from build123d import *

# Parameters (mm, degrees)
MODEL_R                 = 8
SALIENTE_EXTRUIR1_DEPTH = 3


with BuildPart() as part:
    # Model → Saliente-Extruir1 (new body)
    with BuildSketch(Plane.XY):
        with BuildLine():
            Line((25.103364369, 60.449776828), (25.103364369, 55.560048431))
            Line((25.103364369, 55.560048431), (25.103364369, -26.439158767))
            ThreePointArc((25.103364369, -26.439158767), (22.813551952, -32.073921627), (17.210031036, -34.439158767))
            Line((17.210031036, -34.439158767), (17.077324369, -34.439158767))
            Line((17.077324369, -34.439158767), (17.077324369, -36.439158767))
            Line((17.077324369, -36.439158767), (17.077324369, -37.439158767))
            Line((17.077324369, -37.439158767), (9.634620202, -37.439158767))
            ThreePointArc((9.634620202, -37.439158767), (8.940767121, -37.73835668), (8.658097702, -38.439105914))
            Line((8.658097702, -38.439105914), (8.658097702, -53.106951569))
            ThreePointArc((8.658097702, -53.106951569), (8.944324254, -53.811296927), (9.644764369, -54.106951569))
            Line((9.644764369, -54.106951569), (16.090657702, -54.106951569))
            ThreePointArc((16.090657702, -54.106951569), (16.791097817, -54.402606212), (17.077324369, -55.106951569))
            Line((17.077324369, -55.106951569), (17.077324369, -61.439951569))
            ThreePointArc((17.077324369, -61.439951569), (16.791097817, -62.144296927), (16.090657702, -62.439951569))
            Line((16.090657702, -62.439951569), (5.154444792, -62.439951569))
            Line((5.154444792, -62.439951569), (5.154444792, -58.439951569))
            Line((5.154444792, -58.439951569), (2.194444792, -58.439951569))
            Line((2.194444792, -58.439951569), (2.194444792, -62.439951569))
            Line((2.194444792, -62.439951569), (-2.852355631, -62.439951569))
            Line((-2.852355631, -62.439951569), (-2.852355631, -34.439951569))
            Line((-2.852355631, -34.439951569), (-11.074248964, -34.439951569))
            Line((-11.074248964, -34.439951569), (-11.074248964, -62.439951569))
            Line((-11.074248964, -62.439951569), (-15.565555208, -62.439951569))
            Line((-15.565555208, -62.439951569), (-15.565555208, -58.439951569))
            Line((-15.565555208, -58.439951569), (-18.525555208, -58.439951569))
            Line((-18.525555208, -58.439951569), (-18.525555208, -62.439951569))
            Line((-18.525555208, -62.439951569), (-30.017262298, -62.439951569))
            ThreePointArc((-30.017262298, -62.439951569), (-30.717702412, -62.144296927), (-31.003928964, -61.439951569))
            Line((-31.003928964, -61.439951569), (-31.003928964, -55.106951569))
            ThreePointArc((-31.003928964, -55.106951569), (-30.717702412, -54.402606212), (-30.017262298, -54.106951569))
            Line((-30.017262298, -54.106951569), (-23.571368964, -54.106951569))
            ThreePointArc((-23.571368964, -54.106951569), (-22.87092885, -53.811296927), (-22.584702298, -53.106951569))
            Line((-22.584702298, -53.106951569), (-22.584702298, -38.439951569))
            ThreePointArc((-22.584702298, -38.439951569), (-22.87092885, -37.735606212), (-23.571368964, -37.439951569))
            Line((-23.571368964, -37.439951569), (-31.003928964, -37.439951569))
            Line((-31.003928964, -37.439951569), (-31.003928964, -34.439951569))
            Line((-31.003928964, -34.439951569), (-31.136635631, -34.439951569))
            ThreePointArc((-31.136635631, -34.439951569), (-36.740156547, -32.074714429), (-39.029968964, -26.439951569))
            Line((-39.029968964, -26.439951569), (-39.029968964, 60.449776828))
            ThreePointArc((-39.029968964, 60.449776828), (-11.813715639, 88.05803587), (22.36143002, 69.755035253))
            ThreePointArc((22.36143002, 69.755035253), (24.083000637, 65.205716618), (25.103364369, 60.449776828))
        make_face()
        with Locations((5.510677067, 59.135571807)):
            Circle(MODEL_R, mode=Mode.SUBTRACT)
        with Locations((-20.142656266, 59.135571807)):
            Circle(MODEL_R, mode=Mode.SUBTRACT)
        Polygon((8.30541929, 8.146386979), (-6.981247377, 8.146386979), (-23.267914044, 8.146386979), (-23.267914044, -23.853613021), (8.30541929, -23.853613021), align=None, mode=Mode.SUBTRACT)
        with BuildLine():
            ThreePointArc((3.470031036, 23.560048431), (5.034204267, 23.261828431), (6.524349919, 23.823111786))
            ThreePointArc((6.524349919, 23.823111786), (-7.083808204, 17.640131856), (-20.962959728, 23.188137015))
            ThreePointArc((-20.962959728, 23.188137015), (-18.18444232, 22.468056811), (-15.529968964, 23.560048431))
            ThreePointArc((-15.529968964, 23.560048431), (-12.029968964, 22.540846026), (-8.529968964, 23.560048431))
            ThreePointArc((-8.529968964, 23.560048431), (-5.029968964, 22.540846026), (-1.529968964, 23.560048431))
            ThreePointArc((-1.529968964, 23.560048431), (0.970031036, 22.144572483), (3.470031036, 23.560048431))
        make_face(mode=Mode.SUBTRACT)
    extrude(amount=SALIENTE_EXTRUIR1_DEPTH)


solid = part.part
Design review of the part built by this model. Coordinates are the model's own, in mm. A direction names the side the tool comes from. Give positions to 0.01 mm unless a question says otherwise; leave off trailing zeros. Order: outer loops, then holes, each group sorted by start corner. A loop starts at its lowest first (then second) coordinate and runs counter-clockwise, first axis right, second up. Notation, with made-up numbers: (58, 45) - (72, 45) arc R26 ccw to (72, 80) - close; hole circle Ø11 at (-24.75, 77.5). An arc over 180 degrees is marked (long way). Write item = value, one per line. Start each with the question number.
Q1. We need section C-C on y = 20. State the section outline as (x, z) points, plus the area to 3 significant figures.
Q2. Mouldability with a two-part tool opening along Y and no side actions: class faces 1 (the face through (-2.852, -49, 1)), 2 (the face through (9.202, 52.038, 1.479)), 3 (the face through (0, -62.44, 1)), 4 (the face through (-18.225, 22.465, 1.479)) as released by +Y, released by -Y, zero draft, split by the parting line, or undercut.
Q3. Clearance check with flat-ended pins moving along their axes: pin 1 Ø0.9 at (y, z) = (-48.5, 1) entering from -X; pin 2 Ø0.9 at (y, z) = (-58.5, 2) entering from -X; pin 3 Ø0.9 at (x, z) = (-5.5, 2) entering from -Y. State where each tip first meets the part, or that it passes through.
Q4. We need section A-A on y = -5. State the section outline as (x, z) points.
Q5. Tool access review of faces 5 (the face through (5.154, -60, 1)), 6 (the face through (8.658, -46, 1)), 7 (the face through (-8, 8.146, 1)): name each direction out of +Z, -Z, +X, -X, +Y, -Y from which nothing blocks a thin tool from reaching the whole face with its end or side.
Q6. To check wall thickness, follow L1, parallel to Y at x = -1, z = 0.7; L2, parallel to Y at x = -5.5, z = 2.3; L3, parallel to Y at x = -11.5, z = 1.2. State the ranges of each line that lie inside material, in increasing order. Write a range as from..to.
Q7. We need section D-D on z = 1.9. State how many separate pieces and enclosed holes the cut face has, plus the area to 3 significant figures.
Q8. We need section B-B on x = -7. State the section outline as (y, z) points, plus the area to 3 significant figures.
Working result:
q1.outline = (-39.03, 0) - (-16.71, 0) - (-16.71, 3) - (-39.03, 3) - close; (1.67, 0) - (25.1, 0) - (25.1, 3) - (1.67, 3) - close
q1.area = 137 mm²
q2.face_1 = zero draft
q2.face_2 = undercut
q2.face_3 = released by -Y
q2.face_4 = undercut
q3.pin_1 = -22.58
q3.pin_2 = -31
q3.pin_3 = -34.44
q4.outline = (-39.03, 0) - (-23.27, 0) - (-23.27, 3) - (-39.03, 3) - close; (8.31, 0) - (25.1, 0) - (25.1, 3) - (8.31, 3) - close
q5.face_5 = +Z, -Z, -Y
q5.face_6 = +Z, -Z, +X
q5.face_7 = +Z, -Z
q6.L1 = -62.44..-23.85, 8.15..18.79, 22.91..54.49, 63.78..87.87
q6.L2 = -34.44..-23.85, 8.15..17.74, 22.56..88.39
q6.L3 = -62.44..-23.85, 8.15..18.05, 22.56..88.1
q7.separate_pieces = 1
q7.enclosed_holes = 4
q7.area = 6,730 mm²
q8.outline = (-34.44, 0) - (-23.85, 0) - (-23.85, 3) - (-34.44, 3) - close; (8.15, 0) - (17.64, 0) - (17.64, 3) - (8.15, 3) - close; (22.85, 0) - (88.42, 0) - (88.42, 3) - (22.85, 3) - close
q8.area = 257 mm²
